from build123d import *

# Parameters (mm, degrees)
SZKIC1_R                    = 10
DODANIE_WYCI_GNI_CIE1_DEPTH = 10
SZKIC2_R                    = 1.6
WYTNIJ_WYCI_GNI_CIE1_DEPTH  = 10


with BuildPart() as part:
    # Szkic1 → Dodanie-wyciągnięcie1 (new body)
    with BuildSketch(Plane.XY):
        Polygon((0, 0), (66, 0), (66, 13.1), (62, 17.886908539), (62, 32.313091461), (66, 37.1), (66, 50.2), (0, 50.2), (0, 37.1), (4, 32.313091461), (4, 17.886908539), (0, 13.1), align=None)
        with Locations((32.952408039, 25.1)):
            Circle(SZKIC1_R, mode=Mode.SUBTRACT)
    extrude(amount=DODANIE_WYCI_GNI_CIE1_DEPTH)

    # Szkic2 → Wytnij-wyciągnięcie1 (cut)
    with BuildSketch(Plane(origin=(0, 50.2, 0), x_dir=(1, 0, 0), z_dir=(0, 1, 0))):
        with Locations(Location((4, -5, 0), (0, 0, 270))):
            Circle(SZKIC2_R)
        with Locations(Location((62, -5, 0), (0, 0, 90))):
            Circle(SZKIC2_R)
    wytnij_wyci_gni_cie1 = extrude(amount=-WYTNIJ_WYCI_GNI_CIE1_DEPTH, mode=Mode.SUBTRACT)

    # Lustro1: Wytnij-wyciągnięcie1 across plane
    add(wytnij_wyci_gni_cie1.mirror(Plane.ZX.offset(25.1)), mode=Mode.SUBTRACT)


solid = part.part
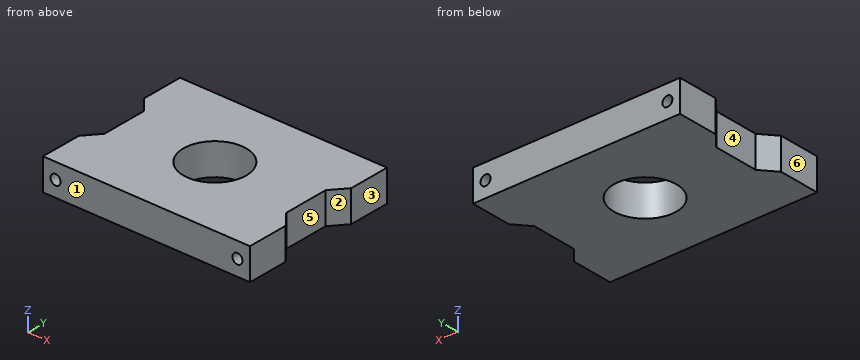
The model under review builds one solid part; all positions refer to its coordinate system, in mm. Face numbers are marked on the shaded views. A direction names the side the tool comes from. Round coordinates to 2 decimals unless told otherwise and drop trailing zeros. Loops run counter-clockwise (first coordinate to the right, second up) from the corner with the lowest first, then second, coordinate; pieces in that order, holes last. Notation, with made-up numbers: M 24,40 L 37,40 A27 cw 37,61 Z; hole C -34.75,-36 d7. An arc over 180 degrees is marked long. Answer as CSV lines item,"result".
1. We need section D-D (x = 31). Give the boundary of the cut face in (y, z).
Outcome:
outline,"M 0,0 L 15.29,0 L 15.29,10 L 0,10 Z; M 34.91,0 L 50.2,0 L 50.2,10 L 34.91,10 Z"
2. To check wall thickness, follow L1, parallel to X at y = 4, z = 5; L2, parallel to Z at x = 62, y = 42.25; L3, parallel to Y at x = 34.5, z = 5. State the ranges of each line that lie inside material, in increasing order. Write a range as [from, to].
Outcome:
L1,"x = [0, 2.4], [5.6, 60.4], [63.6, 66]"
L2,"z = [0, 3.4], [6.6, 10]"
L3,"y = [0, 15.22], [34.98, 50.2]"
3. Insertion check: pin 1 Ø2.5 at (x, z) = (61.5, 5) entering from +Y; pin 2 Ø3 at (x, z) = (62, 5) entering from +Y; pin 3 Ø2.5 at (x, z) = (4, 5) entering from -Y; pin 4 Ø3 at (y, z) = (24.5, 4.5) entering from +X. Each pin has a flat end and moves straight along its axis. Give the tip position at first contact, or say it passes through.
Outcome:
pin 1,"stops at y = 50.2"
pin 2,"stops at y = 40.2"
pin 3,"stops at y = 10"
pin 4,"stops at x = 62"
4. We need section B-B (y = 44). Give the boundary of the cut face in (x, z), plus the area to 3 significant figures.
Outcome:
outline,"M 0,0 L 66,0 L 66,10 L 0,10 Z; hole C 4,5 d3.2; hole C 62,5 d3.2"
area,"644 mm2"
5. Draft analysis for pull direction Y (two halves, no side actions). For the marked faces 1, 2 and 3, state which applies: pulls with the +Y half, pulls with the -Y half, needs draft (parallel to the pull), parting line crosses it, or undercut.
Outcome:
face 1,"pulls with the -Y half"
face 2,"undercut"
face 3,"needs draft"
6. For the marked faces 4, 5 and 6, list the 3-axis set-ups (+Z, -Z, +X, -X, +Y, -Y) from which the entire face can be reached by the end or side of a thin tool; tool diameter is ignored.
Outcome:
face 4,"+Z, -Z, -X"
face 5,"+Z, -Z, +X"
face 6,"+Z, -Z, -X, +Y, -Y"
7. We need section A-A (y = 25.1). Give the boundary of the cut face in (x, z), plus the area to 3 significant figures.
Outcome:
outline,"M 4,0 L 22.95,0 L 22.95,10 L 4,10 Z; M 42.95,0 L 62,0 L 62,10 L 42.95,10 Z"
area,"380 mm2"
